Build history of the part. All positions in model axes, mm. A direction names the side the tool comes from. Give positions to 0.01 mm unless a question says otherwise; leave off trailing zeros. Order: outer loops, then holes, each group sorted by start corner. A loop starts at its lowest first (then second) coordinate and runs counter-clockwise, first axis right, second up. Notation, with made-up numbers: (88, 40.5) - (108, 40.5) arc R13 ccw to (108, 54.5) - close; hole circle Ø10 at (27.5, 88.5). An arc over 180 degrees is marked (long way). One line per item, written item: value.
```python
from build123d import *

# Parameters (mm, degrees)
EXTRUDE_1_DEPTH     = 2
FILLET_1_R          = 2
SKETCH_2_W          = 35.782546262
SKETCH_2_H          = 59.110257758
CUT_EXTRUDE_1_DEPTH = 1
FILLET_2_R          = 1


with BuildPart() as part:
    # 草图1 → 凸台-拉伸1 (new body)
    with BuildSketch(Plane(origin=(0, 0, 0), x_dir=(1, 0, 0), z_dir=(0, 1, 0))):
        with BuildLine():
            Line((-8.359432933, 36.099160402), (13.140567067, 36.099160402))
            ThreePointArc((13.140567067, 36.099160402), (14.554780629, 35.513373964), (15.140567067, 34.099160402))
            Line((15.140567067, 34.099160402), (15.140567067, -14.400839598))
            ThreePointArc((15.140567067, -14.400839598), (14.554780629, -15.81505316), (13.140567067, -16.400839598))
            Line((13.140567067, -16.400839598), (-8.359432933, -16.400839598))
            ThreePointArc((-8.359432933, -16.400839598), (-9.773646496, -15.81505316), (-10.359432933, -14.400839598))
            Line((-10.359432933, -14.400839598), (-10.359432933, 34.099160402))
            ThreePointArc((-10.359432933, 34.099160402), (-9.773646496, 35.513373964), (-8.359432933, 36.099160402))
        make_face()
        with BuildLine():
            Line((-6.609432933, 16.136804798), (-6.609432933, -4.363195202))
            ThreePointArc((-6.609432933, -4.363195202), (2.390567067, -5.863195202), (11.390567067, -4.363195202))
            Line((11.390567067, -4.363195202), (11.390567067, 16.136804798))
            ThreePointArc((11.390567067, 16.136804798), (8.754528097, 22.500765829), (2.390567067, 25.136804798))
            ThreePointArc((2.390567067, 25.136804798), (-3.973393964, 22.500765829), (-6.609432933, 16.136804798))
        make_face(mode=Mode.SUBTRACT)
    extrude(amount=EXTRUDE_1_DEPTH)

    # 圆角1
    fillet_1_edges = [part.edges().sort_by_distance(p)[0] for p in [
        (-9.773646496, 2, 15.81505316),
        (2.390567067, 2, 16.400839598),
        (14.554780629, 2, 15.81505316),
        (15.140567067, 2, -9.849160402),
        (-9.773646496, 2, -35.513373964),
        (14.554780629, 2, -35.513373964),
        (2.390567067, 2, -36.099160402),
        (-10.359432933, 2, -9.849160402),
    ]]
    fillet(fillet_1_edges, radius=FILLET_1_R - 0.0001)  # a hair under: the kernel refuses the full size

    # 草图2 → 切除-拉伸1 (cut)
    with BuildSketch(Plane(origin=(0, 0, 0), x_dir=(-1, 0, 0), z_dir=(0, -1, 0))):
        with Locations((0.496790494, 10.685635763)):
            Rectangle(SKETCH_2_W, SKETCH_2_H)
    extrude(amount=-CUT_EXTRUDE_1_DEPTH, mode=Mode.SUBTRACT)

    # 圆角2
    fillet_2_edges = [part.edges().sort_by_distance(p)[0] for p in [
        (11.390567067, 2, -5.886804798),
        (2.390567067, 2, -25.136804798),
        (-6.609432933, 2, -5.886804798),
        (2.390567067, 2, 5.863195202),
    ]]
    fillet(fillet_2_edges, radius=FILLET_2_R - 0.0001)  # a hair under: the kernel refuses the full size


solid = part.part
```
(1) Drill centre lines: line 1 (Z direction, x = -3.25, y = 1.8); line 2 (Z direction, x = 4.75, y = 1.1); line 3 (X direction, y = 1.15, z = -1). Where is each one in solid material? Low to high.
Completed:
line 1: -34.97 to -23.66, 5.69 to 15.27
line 2: -35.77 to -24.83, 5.77 to 16.07
line 3: -10 to -6.62, 11.4 to 14.78
(2) Slice it at B-B, the plane z = -28. Give the cut face in (x, y), and give its area (3 significant figures).
Completed:
outline: (-10.09, 1) - (14.87, 1) arc R2 ccw to (13.14, 2) - (-8.36, 2) arc R2 ccw to start
area: 24.0 mm²
(3) 3-axis set-ups, long thin cutter, end or side, ignore diameter. For faces 1 (the face through (14.153, 1.725, -9.51)), 2 (the face through (-6.91, 1.715, -5.386)): which of +Z, -Z, +X, -X, +Y, -Y reach the whole face in a straight line?
Completed:
face 1: +Z, -Z, +X, +Y
face 2: +Y
(4) Pull direction Z, two halves, no side cores. Call faces 3 (the face through (11.691, 1.715, -5.683)), 4 (the face through (2.541, 1.725, -35.112)), 5 (the face through (14, 1, -10)): +Z half, -Z half, draft (parallel to the pull), parting line (faces both ways), or undercut.
Completed:
face 3: undercut
face 4: -Z half
face 5: draft
